```python
from build123d import *

# Parameters (mm, degrees)
SKETCH1_R           = 15
BOSS_EXTRUDE1_DEPTH = 100
SKETCH2_R           = 7.5
CUT_EXTRUDE1_DEPTH  = 130
SKETCH3_W           = 23.300503328
SKETCH3_H           = 40
SKETCH3_R           = 5
BOSS_EXTRUDE2_DEPTH = 7.5


with BuildPart() as part:
    # Sketch1 → Boss-Extrude1 (new body)
    with BuildSketch(Plane.XY):
        Circle(SKETCH1_R)
    extrude(amount=BOSS_EXTRUDE1_DEPTH)

    # Sketch2 → Cut-Extrude1 (cut)
    with BuildSketch(Plane.XY.offset(100)):
        Circle(SKETCH2_R)
    extrude(amount=-CUT_EXTRUDE1_DEPTH, mode=Mode.SUBTRACT)

    # Sketch3 → Boss-Extrude2 (add, symmetric)
    with BuildSketch(Plane(origin=(0, 0, 0), x_dir=(1, 0, 0), z_dir=(0, 1, 0))):
        Rectangle(SKETCH3_W, SKETCH3_H)
        with Locations((0, 10)):
            Circle(SKETCH3_R, mode=Mode.SUBTRACT)
    extrude(amount=BOSS_EXTRUDE2_DEPTH, both=True)


solid = part.part
```
Verification items for the finished model (mm, model axes). A direction names the side the tool comes from. Round coordinates to 2 decimals unless told otherwise and drop trailing zeros. Write each loop counter-clockwise with the first axis right and the second up, starting at its lowest first coordinate (ties: lowest second). Pieces come first, ordered by that corner, then holes.
1. Gauge pin test, flat ends, axial feed: P1, Ø6, axis at x = 4.5, z = -9.5, coming from the +Y side; P2, Ø16, axis at x = -2, z = -5.5, coming from the -Y side; P3, Ø6, axis at x = 4, z = 61, coming from the +Y side; P4, Ø3, axis at x = 11, z = 47.5, coming from the +Y side. Record the tip position at first contact, or that the pin passes through.
2. Section check C-C on y = 0. Enter the section's corners in (x, z).
3. Draft check along Z on faces 1 (the flat face through (0, 0, -20)), 2 (the flat face through (0, 0, 20)), 3 (the cylindrical face through (-0.651, -0.105, -14.957)), 4 (the cylindrical face through (-14.985, 0.66, 49.3)). Enter one of: +Z half, -Z half, draft (parallel to the pull), parting line (faces both ways), or undercut.
4. Section check A-A on x = 0. Enter the section's corners in (y, z), plus the area to 3 significant figures.
5. Scan lines: L1, parallel to X at y = -4, z = -10; L2, parallel to Y at x = 0, z = 73.5; L3, parallel to X at y = -6, z = -11.5. Record each from-to range of solid material in increasing order.
6. Section check D-D on x = -9. Enter the section's corners in (y, z).
7. Section check B-B on z = -10. Enter the section's corners in (x, y).
8. Access from +Z, -Z, +X, -X, +Y, -Y to the whole of each face (thin tool, end or side, straight path). Record for faces 5 (the flat face through (-11.65, 0, -10)), 6 (the flat face through (11.65, 0, -10)), 7 (the cylindrical face through (-7.493, 0.33, 60.56)).
Answer:
1. P1: stops at y = 7.5
1. P2: stops at y = -15
1. P3: stops at y = 14.97
1. P4: stops at y = 11.61
2. outline: (-15, 0) - (-11.65, 0) - (-11.65, -20) - (11.65, -20) - (11.65, 0) - (15, 0) - (15, 100) - (7.5, 100) - (7.5, 20) - (-7.5, 20) - (-7.5, 100) - (-15, 100) - close; hole circle Ø10 at (0, -10)
3. face 1: -Z half
3. face 2: +Z half
3. face 3: undercut
3. face 4: draft
4. outline: (-15, 0) - (-7.5, 0) - (-7.5, -5) - (7.5, -5) - (7.5, 0) - (15, 0) - (15, 100) - (7.5, 100) - (7.5, 20) - (-7.5, 20) - (-7.5, 100) - (-15, 100) - close; (-7.5, -20) - (7.5, -20) - (7.5, -15) - (-7.5, -15) - close
4. area: 1,950 mm2
5. L1: x = -11.65 to -5, 5 to 11.65
5. L2: y = -15 to -7.5, 7.5 to 15
5. L3: x = -11.65 to -4.77, 4.77 to 11.65
6. outline: (-12, 0) - (-7.5, 0) - (-7.5, -20) - (7.5, -20) - (7.5, 0) - (12, 0) - (12, 100) - (-12, 100) - close
7. outline: (-11.65, -7.5) - (-5, -7.5) - (-5, 7.5) - (-11.65, 7.5) - close; (5, -7.5) - (11.65, -7.5) - (11.65, 7.5) - (5, 7.5) - close
8. face 5: -Z, -X, +Y, -Y
8. face 6: -Z, +X, +Y, -Y
8. face 7: +Z
